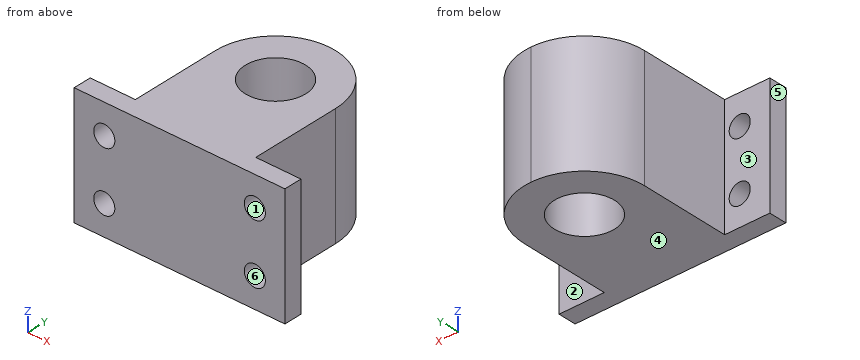
```python
from build123d import *

# Parameters (mm, degrees)
SKETCH_1_W          = 35
SKETCH_1_H          = 3
SKETCH_1_W_2        = 20
SKETCH_1_H_2        = 25
EXTRUDE_1_DEPTH     = 20
FILLET_1_R          = 10
FILLET_2_R          = 10
CUT_EXTRUDE_1_REACH = 51.082
SKETCH_2_R          = 5
CUT_EXTRUDE_2_REACH = 49.434
SKETCH_4_R          = 1.75


with BuildPart() as part:
    # 草图1 → 凸台-拉伸1 (new body)
    with BuildSketch(Plane.XY):
        with Locations((17.5, 1.5)):
            Rectangle(SKETCH_1_W, SKETCH_1_H)
        with Locations((17.5, 15.5)):
            Rectangle(SKETCH_1_W_2, SKETCH_1_H_2)
    extrude(amount=EXTRUDE_1_DEPTH)

    # 圆角1
    fillet_1_edges = [part.edges().sort_by_distance(p)[0] for p in [
        (27.5, 28, 10),
    ]]
    fillet(fillet_1_edges, radius=FILLET_1_R)

    # 圆角2
    fillet_2_edges = [part.edges().sort_by_distance(p)[0] for p in [
        (7.5, 28, 10),
    ]]
    fillet(fillet_2_edges, radius=FILLET_2_R - 0.0001)  # a hair under: the kernel refuses the full size

    # 草图2 → 切除-拉伸1 (cut, up to next)
    with BuildSketch(Plane.XY.offset(20), mode=Mode.PRIVATE) as cut_extrude_1_sk1:
        with Locations((17.5, 18)):
            Circle(SKETCH_2_R)
    cut_extrude_1_tool1 = extrude(cut_extrude_1_sk1.sketch, amount=-CUT_EXTRUDE_1_REACH, mode=Mode.PRIVATE) & part.part
    add(cut_extrude_1_tool1.solids().sort_by_distance((17.5, 18, 20))[0], mode=Mode.SUBTRACT)

    # 草图4 → 切除-拉伸2 (cut, up to next)
    with BuildSketch(Plane(origin=(0, 3, 0), x_dir=(1, 0, 0), z_dir=(0, 1, 0)), mode=Mode.PRIVATE) as cut_extrude_2_sk1:
        with Locations(Location((30, -15, 0), (0, 0, 270))):
            Circle(SKETCH_4_R)
    cut_extrude_2_tool1 = extrude(cut_extrude_2_sk1.sketch, amount=-CUT_EXTRUDE_2_REACH, mode=Mode.PRIVATE) & part.part
    # 草图4 → 切除-拉伸2 (cut, up to next)
    with BuildSketch(Plane(origin=(0, 3, 0), x_dir=(1, 0, 0), z_dir=(0, 1, 0)), mode=Mode.PRIVATE) as cut_extrude_2_sk2:
        with Locations(Location((30, -5, 0), (0, 0, 270))):
            Circle(SKETCH_4_R)
    cut_extrude_2_tool2 = extrude(cut_extrude_2_sk2.sketch, amount=-CUT_EXTRUDE_2_REACH, mode=Mode.PRIVATE) & part.part
    # 草图4 → 切除-拉伸2 (cut, up to next)
    with BuildSketch(Plane(origin=(0, 3, 0), x_dir=(1, 0, 0), z_dir=(0, 1, 0)), mode=Mode.PRIVATE) as cut_extrude_2_sk3:
        with Locations(Location((5, -15, 0), (0, 0, 270))):
            Circle(SKETCH_4_R)
    cut_extrude_2_tool3 = extrude(cut_extrude_2_sk3.sketch, amount=-CUT_EXTRUDE_2_REACH, mode=Mode.PRIVATE) & part.part
    # 草图4 → 切除-拉伸2 (cut, up to next)
    with BuildSketch(Plane(origin=(0, 3, 0), x_dir=(1, 0, 0), z_dir=(0, 1, 0)), mode=Mode.PRIVATE) as cut_extrude_2_sk4:
        with Locations(Location((5, -5, 0), (0, 0, 270))):
            Circle(SKETCH_4_R)
    cut_extrude_2_tool4 = extrude(cut_extrude_2_sk4.sketch, amount=-CUT_EXTRUDE_2_REACH, mode=Mode.PRIVATE) & part.part
    add(cut_extrude_2_tool1.solids().sort_by_distance((30, 3, 15))[0], mode=Mode.SUBTRACT)
    add(cut_extrude_2_tool2.solids().sort_by_distance((30, 3, 5))[0], mode=Mode.SUBTRACT)
    add(cut_extrude_2_tool3.solids().sort_by_distance((5, 3, 15))[0], mode=Mode.SUBTRACT)
    add(cut_extrude_2_tool4.solids().sort_by_distance((5, 3, 5))[0], mode=Mode.SUBTRACT)


solid = part.part
```
CAD build for the part. Positions are in the model's coordinates, mm. Face numbers are marked on the shaded views. A direction names the side the tool comes from. Round coordinates to 2 decimals unless told otherwise and drop trailing zeros. Loops run counter-clockwise (first coordinate to the right, second up) from the corner with the lowest first, then second, coordinate; pieces in that order, holes last. Notation, with made-up numbers: M -5,-6.75 L 43,-6.75 A14 ccw 43,5.25 Z; hole C 23,24 d6. An arc over 180 degrees is marked long. Use a Markdown table: item, result. Add a question column.
(1) Cut at C-C (x = 30). Give the cut face in (y, z), and give its area (3 significant figures).
(2) Flat gauge pins, fed straight in: pin 1 (4.5 mm diameter, centred on y = 9.5, z = 5.5, fed in from +X); pin 2 (2 mm diameter, centred on x = 30, z = 5, fed in from -Y); pin 3 (3 mm diameter, centred on y = 20.5, z = 9.5, fed in from -X); pin 4 (4.5 mm diameter, centred on y = 10.5, z = 8, fed in from -X). Where does each tip first touch, or does it go through?
(3) Pull direction Z, two halves, no side cores. Call the marked faces 4, 5 and 6: +Z half, -Z half, draft (parallel to the pull), parting line (faces both ways), or undercut.
(4) Which spindle directions (+Z, -Z, +X, -X, +Y, -Y) get a long thin tool onto all of the face, cutting with end or side? Do the marked faces 1, 2 and 3. Say none if no direction does.
(5) Drill centre lines: line 1 (Y direction, x = 17.5, z = 8); line 2 (X direction, y = 4.5, z = 13.25); line 3 (Y direction, x = 4, z = 1.75). Where is each one in solid material? Low to high.
(6) Cut at A-A (z = 5). State how many separate pieces and enclosed holes the cut face has, and give its area (3 significant figures).
(7) Cut at D-D (y = 17.25). Give the cut face in (x, z).
Geometry says:
| question | item | result |
|---|---|---|
| 1 | outline | M 0,0 L 3,0 L 3,3.25 L 0,3.25 Z; M 0,6.75 L 3,6.75 L 3,13.25 L 0,13.25 Z; M 0,16.75 L 3,16.75 L 3,20 L 0,20 Z |
| 1 | area | 39.0 mm² |
| 2 | pin 1 | stops at x = 27.5 |
| 2 | pin 2 | passes through |
| 2 | pin 3 | stops at x = 7.55 |
| 2 | pin 4 | stops at x = 7.5 |
| 3 | face 4 | -Z half |
| 3 | face 5 | draft |
| 3 | face 6 | undercut |
| 4 | face 1 | +Y, -Y |
| 4 | face 2 | +Z, -Z, +X, +Y |
| 4 | face 3 | +Z, -Z, -X, +Y |
| 5 | line 1 | y = 0 to 13, 23 to 28 |
| 5 | line 2 | x = 7.5 to 27.5 |
| 5 | line 3 | y = 0 to 3 |
| 6 | separate pieces | 3 |
| 6 | enclosed holes | 1 |
| 6 | area | 463 mm² |
| 7 | outline | M 7.5,0 L 12.56,0 L 12.56,20 L 7.5,20 Z; M 22.44,0 L 27.5,0 L 27.5,20 L 22.44,20 Z |
